CAD build for the part. Positions are in the model's coordinates, mm. Face numbers are marked on the shaded views. A direction names the side the tool comes from. Give positions to 0.01 mm unless a question says otherwise; leave off trailing zeros. Write each loop counter-clockwise with the first axis right and the second up, starting at its lowest first coordinate (ties: lowest second). Pieces come first, ordered by that corner, then holes. Notation, with made-up numbers: (17.25, 25) - (70.25, 25) arc R24 cw to (70.25, 56) - close; hole circle Ø5 at (-11.75, 14). An arc over 180 degrees is marked (long way). Answer as a JSON object with one key per item and string values.
from build123d import *

# Parameters (mm, degrees)
SKIZZE1_W                                = 75
SKIZZE1_H                                = 60
AUFSATZ_LINEAR_AUSTRAGEN1_DEPTH          = 25
WANDUNG1_T                               = -2
VERRUNDUNG1_R                            = 5
SKIZZE2_W                                = 9.2
SKIZZE2_H                                = 13
SCHNITT_LINEAR_AUSTRAGEN1_DEPTH          = 25
VERRUNDUNG2_R                            = 1
SKIZZE3_W                                = 10.2
SKIZZE3_H                                = 5.2
SCHNITT_LINEAR_AUSTRAGEN2_DEPTH          = 25
VERRUNDUNG3_R                            = 1
F_3_0_3_DURCHMESSER_BOHRUNG1_D           = 3
F_3_0_3_DURCHMESSER_BOHRUNG1_CSINK_D     = 3.05
F_3_0_3_DURCHMESSER_BOHRUNG1_CSINK_ANGLE = 90
F_2_0_2_DURCHMESSER_BOHRUNG1_D           = 2
F_2_0_2_DURCHMESSER_BOHRUNG1_DEPTH       = 20
F_2_0_2_DURCHMESSER_BOHRUNG1_CSINK_D     = 2.05
F_2_0_2_DURCHMESSER_BOHRUNG1_CSINK_ANGLE = 90
F_2_0_2_DURCHMESSER_BOHRUNG1_TIP         = 0.600860619


with BuildPart() as part:
    # Skizze1 → Aufsatz-Linear austragen1 (new body)
    with BuildSketch(Plane(origin=(0, 0, 0), x_dir=(1, 0, 0), z_dir=(0, 1, 0))):
        Rectangle(SKIZZE1_W, SKIZZE1_H)
    extrude(amount=AUFSATZ_LINEAR_AUSTRAGEN1_DEPTH)

    # Wandung1
    wandung1_openings = [part.faces().sort_by_distance(p)[0] for p in [
        (0, 25, 0),
    ]]
    offset(amount=WANDUNG1_T, openings=wandung1_openings, kind=Kind.INTERSECTION)

    # Verrundung1
    verrundung1_edges = [part.edges().sort_by_distance(p)[0] for p in [
        (35.5, 13.5, 28),
        (35.5, 13.5, -28),
        (-35.5, 13.5, -28),
        (-35.5, 13.5, 28),
        (37.5, 12.5, 30),
        (-37.5, 12.5, 30),
        (-37.5, 12.5, -30),
        (37.5, 12.5, -30),
    ]]
    fillet(verrundung1_edges, radius=VERRUNDUNG1_R)

    # Skizze2 → Schnitt-Linear austragen1 (cut)
    with BuildSketch(Plane(origin=(37.5, 0, 0), x_dir=(0, 0, -1), z_dir=(1, 0, 0))):
        with Locations((18, 11.5)):
            Rectangle(SKIZZE2_W, SKIZZE2_H)
    extrude(amount=-SCHNITT_LINEAR_AUSTRAGEN1_DEPTH, mode=Mode.SUBTRACT)

    # Verrundung2
    verrundung2_edges = [part.edges().sort_by_distance(p)[0] for p in [
        (36.5, 5, -13.4),
        (36.5, 18, -13.4),
        (36.5, 18, -22.6),
        (36.5, 5, -22.6),
    ]]
    fillet(verrundung2_edges, radius=VERRUNDUNG2_R)

    # Skizze3 → Schnitt-Linear austragen2 (cut)
    with BuildSketch(Plane(origin=(37.5, 0, 0), x_dir=(0, 0, -1), z_dir=(1, 0, 0))):
        with Locations((-11.28, 7.1)):
            Rectangle(SKIZZE3_W, SKIZZE3_H)
    extrude(amount=-SCHNITT_LINEAR_AUSTRAGEN2_DEPTH, mode=Mode.SUBTRACT)

    # Verrundung3
    verrundung3_edges = [part.edges().sort_by_distance(p)[0] for p in [
        (36.5, 4.5, 16.38),
        (36.5, 9.7, 16.38),
        (36.5, 9.7, 6.18),
        (36.5, 4.5, 6.18),
    ]]
    fillet(verrundung3_edges, radius=VERRUNDUNG3_R)

    # Ø3.0 (3) Durchmesser Bohrung1 (through all)
    with Locations(Plane(origin=(0, 2, 0), x_dir=(1, 0, 0), z_dir=(0, 1, 0))):
        with Locations((21.546108128, 23.974231713), (-30.532956337, 18.838889879), (-30.532956337, -9.070576608), (20.26227267, -24.309145311)):
            CounterSinkHole(F_3_0_3_DURCHMESSER_BOHRUNG1_D / 2, F_3_0_3_DURCHMESSER_BOHRUNG1_CSINK_D / 2, counter_sink_angle=F_3_0_3_DURCHMESSER_BOHRUNG1_CSINK_ANGLE)

    # Ø2.0 (2) Durchmesser Bohrung1
    with Locations(Plane(origin=(0, 28, 0), x_dir=(1, 0, 0), z_dir=(0, 1, 0))):
        with Locations((-35.165927774, 27.602462356), (35.054289908, 27.602462356), (35.054289908, -27.658281289), (-35.165927774, -27.658281289)):
            CounterSinkHole(F_2_0_2_DURCHMESSER_BOHRUNG1_D / 2, F_2_0_2_DURCHMESSER_BOHRUNG1_CSINK_D / 2, depth=F_2_0_2_DURCHMESSER_BOHRUNG1_DEPTH, counter_sink_angle=F_2_0_2_DURCHMESSER_BOHRUNG1_CSINK_ANGLE)
            with Locations((0, 0, -(F_2_0_2_DURCHMESSER_BOHRUNG1_DEPTH + F_2_0_2_DURCHMESSER_BOHRUNG1_TIP / 2))):  # 118° drill point
                Cone(0, F_2_0_2_DURCHMESSER_BOHRUNG1_D / 2, F_2_0_2_DURCHMESSER_BOHRUNG1_TIP, mode=Mode.SUBTRACT)


solid = part.part
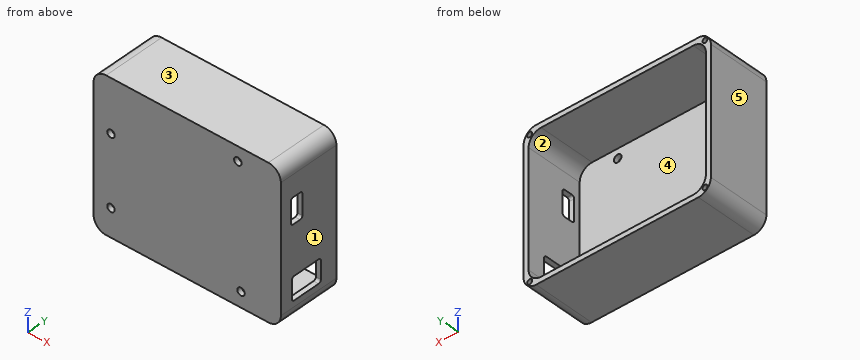
Item 1: Cut at A-A (y = 3.25). Give the cut face in (x, z).
Entries:
{"outline": "(-37.5, -25) arc R5 ccw to (-32.5, -30) - (32.5, -30) arc R5 ccw to (37.5, -25) - (37.5, 25) arc R5 ccw to (32.5, 30) - (-32.5, 30) arc R5 ccw to (-37.5, 25) - close; hole (-35.5, -23) arc R5 ccw to (-30.5, -28) - (30.5, -28) arc R5 ccw to (35.5, -23) - (35.5, 23) arc R5 ccw to (30.5, 28) - (-30.5, 28) arc R5 ccw to (-35.5, 23) - close"}
Item 2: Cut at C-C (x = -26). Give the cut face in (y, z).
Entries:
{"outline": "(0, -30) - (25, -30) - (25, -28) - (2, -28) - (2, 28) - (25, 28) - (25, 30) - (0, 30) - close"}
Item 3: Cut at B-B (z = -8.5). Give the cut face in (x, y).
Entries:
{"outline": "(-37.5, 0) - (37.5, 0) - (37.5, 25) - (35.5, 25) - (35.5, 2) - (-35.5, 2) - (-35.5, 25) - (-37.5, 25) - close"}
Item 4: Mould opens along X. For the marked faces 1, 2 and 3 say: +X half, -X half, draft (parallel to the pull), parting line (faces both ways), or undercut.
Entries:
{"face 1": "+X half", "face 2": "undercut", "face 3": "draft"}
Item 5: Probe line 1 (Z direction, x = -12.5, y = 8.75); line 2 (X direction, y = 7.5, z = 20); line 3 (Y direction, x = 29, z = 26.5). List the from-to ranges inside material, lowest first. Write a range as from..to.
Entries:
{"line 1": "-30..-28, 28..30", "line 2": "-37.5..-35.5, 35.5..37.5", "line 3": "0..2"}
Item 6: Flat gauge pins, fed straight in: P1, Ø3.5, axis at x = -30.53, z = -18.84, coming from the +Y side; P2, Ø1, axis at x = 36, y = 9.5, coming from the +Z side; P3, Ø1.8, axis at x = 20.26, z = 24.31, coming from the -Y side; P4, Ø2, axis at x = 36.5, y = 7.5, coming from the -Z side. Where does each tip first touch, or does it go through?
Entries:
{"P1": "y = 2", "P2": "z = 29", "P3": "through", "P4": "z = -29"}
Item 7: Cut at D-D (y = 20). Give the cut face in (x, z), and give its area (3 significant figures).
Entries:
{"outline": "(-37.5, -25) arc R5 ccw to (-32.5, -30) - (32.5, -30) arc R5 ccw to (37.5, -25) - (37.5, 25) arc R5 ccw to (32.5, 30) - (-32.5, 30) arc R5 ccw to (-37.5, 25) - close; hole circle Ø2 at (-35.17, -27.6); hole circle Ø2 at (-35.17, 27.66); hole (-35.5, -23) arc R5 ccw to (-30.5, -28) - (30.5, -28) arc R5 ccw to (35.5, -23) - (35.5, 23) arc R5 ccw to (30.5, 28) - (-30.5, 28) arc R5 ccw to (-35.5, 23) - close; hole circle Ø2 at (35.05, -27.6); hole circle Ø2 at (35.05, 27.66)", "area": "511 mm2"}
Item 8: Which spindle directions (+Z, -Z, +X, -X, +Y, -Y) get a long thin tool onto all of the face, cutting with end or side? Do the marked faces 4 and 5. Say none if no direction does.
Entries:
{"face 4": "+Y", "face 5": "+Z, -Z, -X, +Y, -Y"}
